Geometry check sheet. Reference: drawing and pictorial views, mm from the part's lowest x, y, z. A direction names the side the tool comes from. Coordinates: 2 decimals unless noted, no trailing zeros. Write each loop counter-clockwise with the first axis right and the second up, starting at its lowest first coordinate (ties: lowest second). Pieces come first, ordered by that corner, then holes. Notation, with made-up numbers: (8, 21) -> (47, 21) arc R15 cw to (47, 43) -> close; hole circle Ø7 at (70.25, 89.5). An arc over 180 degrees is marked (long way). Use a Markdown table: item, result.
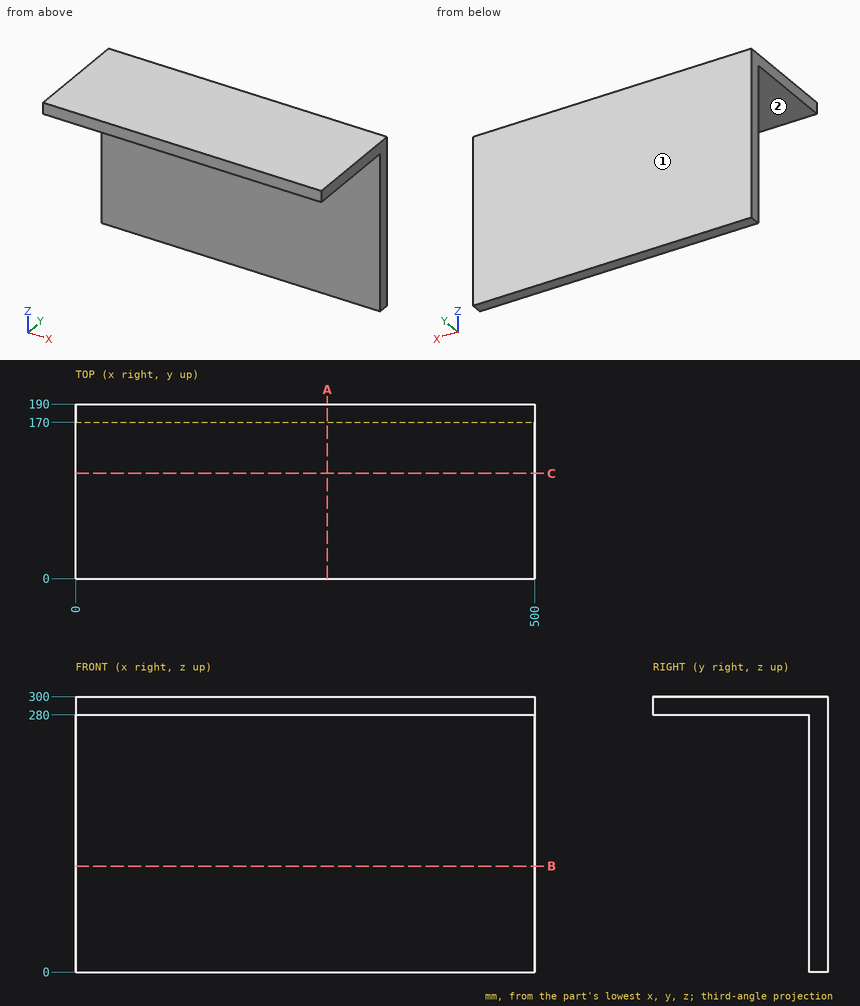
Item 1: Thickness scan on L1, parallel to Z at x = 153, y = 120; L2, parallel to Y at x = 275.5, z = 170. Record the ranges inside material, lowest first. Write a range as [from, to].
Answer block:
| item | result |
|---|---|
| L1 | z = [280, 300] |
| L2 | y = [170, 190] |
Item 2: Section check A-A on x = 274. Record the boundary of the cut face in (y, z), then the cut area to 3 significant figures.
Answer block:
| item | result |
|---|---|
| outline | (0, 280) -> (170, 280) -> (170, 0) -> (190, 0) -> (190, 300) -> (0, 300) -> close |
| area | 9,400 mm^2 |
Item 3: Section check C-C on y = 114.5. Record the boundary of the cut face in (x, z), then the cut area to 3 significant figures.
Answer block:
| item | result |
|---|---|
| outline | (0, 280) -> (500, 280) -> (500, 300) -> (0, 300) -> close |
| area | 10,000 mm^2 |
Item 4: Section check B-B on z = 115.5. Record the boundary of the cut face in (x, y), then the cut area to 3 significant figures.
Answer block:
| item | result |
|---|---|
| outline | (0, 170) -> (500, 170) -> (500, 190) -> (0, 190) -> close |
| area | 10,000 mm^2 |
Item 5: Tool access check on the marked faces 1 and 2. Record the directions out of +Z, -Z, +X, -X, +Y, -Y that give a thin tool (end or side, any length) a straight path to the whole face; none if there is none.
Answer block:
| item | result |
|---|---|
| face 1 | +Z, -Z, +X, -X, +Y |
| face 2 | -Z, +X, -X, -Y |
Item 6: Depth check by flat-ended pin: P1, Ø1, axis at x = 223.5, z = 259.5, coming from the -Y side; P2, Ø4, axis at x = 340.5, y = 50.5, coming from the -Z side. Enter the tip coordinate at first touch or a pass-through.
Answer block:
| item | result |
|---|---|
| P1 | stops at y = 170 |
| P2 | stops at z = 280 |
